Read the model definition and answer for the solid it produces. Units are mm, in the model's axes. Face numbers are marked on the shaded views. A direction names the side the tool comes from. Give positions to 0.01 mm unless a question says otherwise; leave off trailing zeros. Write each loop counter-clockwise with the first axis right and the second up, starting at its lowest first coordinate (ties: lowest second). Pieces come first, ordered by that corner, then holes. Notation, with made-up numbers: (46, 40.5) - (105, 40.5) arc R15 cw to (105, 62.5) - close; hole circle Ø2 at (29.5, -26). An arc over 180 degrees is marked (long way). Answer as CSV lines item,"result".
```python
from build123d import *

# Parameters (mm, degrees)
SKETCH_1_R      = 5.25
SKETCH_1_R_2    = 6
SKETCH_1_R_3    = 1.55
EXTRUDE_1_DEPTH = 7
FILLET_1_R      = 2


with BuildPart() as part:
    # 草图1 → 凸台-拉伸1 (new body)
    with BuildSketch(Plane.XY):
        with BuildLine():
            Line((0, 9.5), (30, 9.5))
            ThreePointArc((30, 9.5), (39.5, 0), (30, -9.5))
            Line((30, -9.5), (0, -9.5))
            ThreePointArc((0, -9.5), (-9.5, 0), (0, 9.5))
        make_face()
        Circle(SKETCH_1_R, mode=Mode.SUBTRACT)
        with Locations((30, 0)):
            Circle(SKETCH_1_R_2, mode=Mode.SUBTRACT)
        with Locations((0, -7)):
            Circle(SKETCH_1_R_3, mode=Mode.SUBTRACT)
        with Locations((-7, 0)):
            Circle(SKETCH_1_R_3, mode=Mode.SUBTRACT)
        with Locations((0, 7)):
            Circle(SKETCH_1_R_3, mode=Mode.SUBTRACT)
        with Locations((7, 0)):
            Circle(SKETCH_1_R_3, mode=Mode.SUBTRACT)
        with BuildLine():
            Line((22.400657923, -6.5), (8.874119675, -6.5))
            ThreePointArc((8.874119675, -6.5), (11, 0), (8.874119675, 6.5))
            Line((8.874119675, 6.5), (22.400657923, 6.5))
            ThreePointArc((22.400657923, 6.5), (20, 0), (22.400657923, -6.5))
        make_face(mode=Mode.SUBTRACT)
    extrude(amount=EXTRUDE_1_DEPTH)

    # 圆角1
    fillet_1_edges = [part.edges().sort_by_distance(p)[0] for p in [
        (22.400657923, -6.5, 3.5),
        (22.400657923, 6.5, 3.5),
        (8.874119675, 6.5, 3.5),
        (8.874119675, -6.5, 3.5),
    ]]
    fillet(fillet_1_edges, radius=FILLET_1_R)


solid = part.part
```
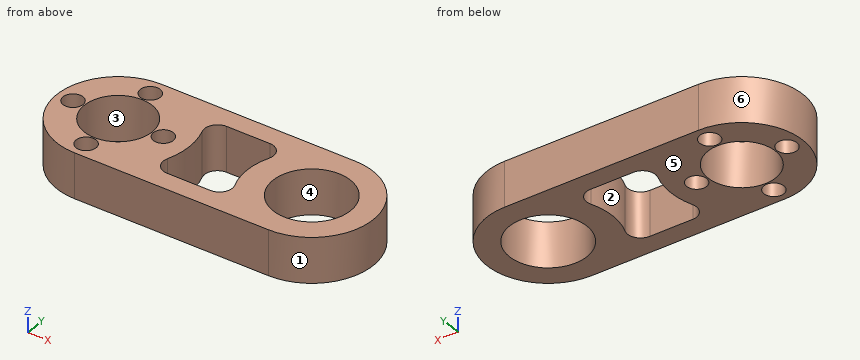
(1) The mould has two halves that part along Y. Classify the marked faces 3, 4, 5 and 6: +Y half, -Y half, draft (parallel to the pull), parting line (faces both ways), or undercut.
Worked out:
face 3,"undercut"
face 4,"undercut"
face 5,"draft"
face 6,"parting line"
(2) This flat-tipped pin is pushed along its axis until it touches: P1, Ø1, axis at y = -7, z = 2.5, coming from the +X side. Where does it stop, or does it pass through?
Worked out:
P1,"stops at x = 36.93"
(3) A cutting plane is placed at B-B (y = 0). Write down the section's boundary in (x, z), and give its area (3 significant figures).
Worked out:
outline,"(-9.5, 0) - (-8.55, 0) - (-8.55, 7) - (-9.5, 7) - close; (-5.45, 0) - (-5.25, 0) - (-5.25, 7) - (-5.45, 7) - close; (5.25, 0) - (5.45, 0) - (5.45, 7) - (5.25, 7) - close; (8.55, 0) - (11, 0) - (11, 7) - (8.55, 7) - close; (20, 0) - (24, 0) - (24, 7) - (20, 7) - close; (36, 0) - (39.5, 0) - (39.5, 7) - (36, 7) - close"
area,"79.1 mm^2"
(4) A cutting plane is placed at A-A (x = 18). Write down the section's boundary in (y, z).
Worked out:
outline,"(-9.5, 0) - (-6.5, 0) - (-6.5, 7) - (-9.5, 7) - close; (6.5, 0) - (9.5, 0) - (9.5, 7) - (6.5, 7) - close"
(5) For the marked faces 1 and 2, determine the directions among +Z, -Z, +X, -X, +Y, -Y from which every point of the face is accessible in a straight line to the end or side of a thin tool.
Worked out:
face 1,"+Z, -Z, +X"
face 2,"+Z, -Z"
(6) Find the intervals of material crossed by L1, parallel to Y at x = 0, z = 5; L2, parallel to Y at x = 30, z = 2; L3, parallel to X at y = -2.75, z = 5.5, in increasing order.
Worked out:
L1,"y = -9.5 to -8.55, -5.45 to -5.25, 5.25 to 5.45, 8.55 to 9.5"
L2,"y = -9.5 to -6, 6 to 9.5"
L3,"x = -9.09 to -4.47, 4.47 to 10.65, 20.39 to 24.67, 35.33 to 39.09"
(7) A cutting plane is placed at D-D (x = 7). Write down the section's boundary in (y, z).
Worked out:
outline,"(-9.5, 0) - (-1.55, 0) - (-1.55, 7) - (-9.5, 7) - close; (1.55, 0) - (9.5, 0) - (9.5, 7) - (1.55, 7) - close"
(8) A cutting plane is placed at C-C (z = 3.25). Write down the section's boundary in (x, y), and give its area (3 significant figures).
Worked out:
outline,"(0, -9.5) - (30, -9.5) arc R9.5 ccw to (30, 9.5) - (0, 9.5) arc R9.5 ccw to start; hole circle Ø3.1 at (-7, 0); hole circle Ø10.5 at (0, 0); hole circle Ø3.1 at (0, -7); hole circle Ø3.1 at (0, 7); hole circle Ø3.1 at (7, 0); hole (10.32, -3.81) arc R2 ccw to (12.2, -6.5) - (18.88, -6.5) arc R2 ccw to (20.73, -3.75) arc R10 cw to (20.73, 3.75) arc R2 ccw to (18.88, 6.5) - (12.2, 6.5) arc R2 ccw to (10.32, 3.81) arc R11 cw to start; hole circle Ø12 at (30, 0)"
area,"498 mm^2"
